Autodesk Inventor part; units mm, degrees
ref_plane "YZ Plane" through (0, 0, 0) normal (1, 0, 0) x (0, 1, 0)
ref_plane "XZ Plane" through (0, 0, 0) normal (0, 1, 0) x (-1, 0, 0)
ref_plane "XY Plane" through (0, 0, 0) normal (0, 0, 1) x (1, 0, 0)
sketch "Sketch1" plane through (0, 0, 0) normal (1, 0, 0) x (0, 1, 0)
  line L0 (0, 0) -> (4.36, 0)
  line L1 (4.36, 0) -> (4.36, 2.025)
  line L2 (4.36, 2.025) -> (4.16, 2.025)
  line L3 (4.16, 2.025) -> (4.16, 2.225)
  line L4 (4.16, 2.225) -> (4.765, 2.225)
  line L5 (4.765, 2.225) -> (4.765, 3.18)
  line L6 (4.765, 3.18) -> (3.44, 3.18)
  line L7 (3.24, 2.98) -> (3.24, 1.27)
  line L8 (3.24, 1.27) -> (0, 1.27)
  line L9 (0, 1.27) -> (0, 0)
  line L10 (3.44, 3.18) -> (3.24, 2.98)
  point P0 (3.24, 3.18)
  dimension "d1" = 8.72
  dimension "d4" = 0.2
  dimension "d5" = 3.18
  dimension "d6" = 9.53
  dimension "d7" = 1.91
  dimension "d8" = 6.48
  dimension "d9" = 0.955
  dimension "d28" = 0.2
  dimension "d29" = 0.2
revolve "Revolution1" add sketch "Sketch1" angle 360 about axis through (0, 0, 1.27) along (0, 0, -1)
hole "Hole1" at (0, 0, 0) direction (0, 0, 1) diameter 3.242 end through all countersink diameter 4.2 countersink angle 120
equation "\"d1\" = C_"
equation "\"d4\" = TD_d"
equation "\"d5\" = A_"
equation "\"d6\" = E_"
equation "\"d7\" = H_"
equation "\"d8\" = B"
equation "\"d9\" = 0.5 * H_"
equation "\"d19\" = 1.05 * NND"
equation "\"A_\" = 3.18"
equation "\"B\" = 6.48"
equation "\"C_\" = 8.72"
equation "\"E_\" = 9.53"
equation "\"H_\" = 1.91"
equation "\"NND\" = 4"
equation "\"TD_d\" = 0.2"
equation "\"Min_Sheet_for_Self_Clinching\" = 1.27"
equation "\"Min_Sheet_for_Flush_Installation\" = 3.18"
equation "\"Min_Dist\" = 8.64"
equation "\"H_Size\" = 8.74"
equation "\"TL\" = 1.27"
properties part number "PR10-M4" material "Stainless Steel"
For this review, take the finished solid that the model builds, in its own axes (mm). Round coordinates to 2 decimals unless told otherwise and drop trailing zeros. Write each loop counter-clockwise with the first axis right and the second up, starting at its lowest first coordinate (ties: lowest second). Pieces come first, ordered by that corner, then holes. Notation, with made-up numbers: (36, 64) - (68, 64) arc R27 cw to (68, 96) - close; hole circle Ø1 at (55.25, 51.5). An arc over 180 degrees is marked (long way). Use CSV: the item, a comma, the result in double quotes.
1) The part is to be moulded in two halves that separate along Y. For faces 1 (the flat face through (-1.4, 1.4, 1.27)), 2 (the cylindrical face through (-3.163, -0.702, 2.113)), 3 (the cylindrical face through (4.256, -0.945, 1.027)), 4 (the flat face through (-4, 2, 2.225)), say which applies: pulls with the +Y half, pulls with the -Y half, needs draft (parallel to the pull), parting line crosses it, or undercut.
Conclusion:
face 1,"undercut"
face 2,"undercut"
face 3,"parting line crosses it"
face 4,"needs draft"
2) Add section C-C on z = 1.9. Write out the cut boundary in (x, y).
Conclusion:
outline,"circle Ø8.72 at (0, 0); hole circle Ø6.48 at (0, 0)"
3) Clearance check with flat-ended pins moving along their axes: pin 1 Ø1.9 at (x, y) = (1.5, 0) entering from +Z; pin 2 Ø1.5 at (y, z) = (2.5, 1) entering from -X; pin 3 Ø4 at (x, y) = (0, 0) entering from -Z. State where each tip first meets the part, or that it passes through.
Conclusion:
pin 1,"stops at z = 1.27"
pin 2,"stops at x = -3.99"
pin 3,"stops at z = 0.06"
4) Wall thickness on line 1 along X through (y, z) = (0, 0.9); line 2 along Y through (x, z) = (1.5, 2.4); line 3 along X through (y, z) = (0.75, 1.6) (3 decimals): over which ranges is each line inside the solid? List them lowest first. Write a range as from..to.
Conclusion:
line 1,"x = -4.36..-1.62, 1.62..4.36"
line 2,"y = -4.52..-2.87, 2.87..4.52"
line 3,"x = -4.295..-3.152, 3.152..4.295"
5) Add section A-A on y = 0. Write out the cut boundary in (x, z) (3 decimals).
Conclusion:
outline,"(-4.765, 2.225) - (-4.16, 2.225) - (-4.16, 2.025) - (-4.36, 2.025) - (-4.36, 0) - (-2.1, 0) - (-1.621, 0.277) - (-1.621, 1.27) - (-3.24, 1.27) - (-3.24, 2.98) - (-3.44, 3.18) - (-4.765, 3.18) - close; (1.621, 0.277) - (2.1, 0) - (4.36, 0) - (4.36, 2.025) - (4.16, 2.025) - (4.16, 2.225) - (4.765, 2.225) - (4.765, 3.18) - (3.44, 3.18) - (3.24, 2.98) - (3.24, 1.27) - (1.621, 1.27) - close"
6) Add section D-D on z = 2.6. Write out the cut boundary in (x, y) (3 decimals), and give its area (3 significant figures).
Conclusion:
outline,"circle Ø9.53 at (0, 0); hole circle Ø6.48 at (0, 0)"
area,"38.4 mm^2"
